from build123d import *

# Parameters (mm, degrees)
EXTRUDE_THIN1_DEPTH = 10
EXTRUDE_THIN1_DRAFT = -10
BOSS_EXTRUDE1_DEPTH = 2
CUT_EXTRUDE1_DEPTH  = 8.123412895
CIRPATTERN1_COUNT   = 4
CUT_EXTRUDE2_DEPTH  = 8.123412895
CIRPATTERN2_COUNT   = 4


with BuildPart() as part:
    # Sketch1 → Extrude-Thin1 (with draft: the straight prism first)
    with BuildSketch(Plane(origin=(0, 0, 0), x_dir=(1, 0, 0), z_dir=(0, 1, 0))):
        with BuildLine():
            ThreePointArc((22.190349254, 3.72), (15.909902577, 15.909902577), (3.72, 22.190349254))
            Line((3.72, 22.190349254), (3.72, 26.21))
            ThreePointArc((3.72, 26.21), (0, 29.93), (-3.72, 26.21))
            Line((-3.72, 26.21), (-3.72, 22.190349254))
            ThreePointArc((-3.72, 22.190349254), (-15.909902577, 15.909902577), (-22.190349254, 3.72))
            Line((-22.190349254, 3.72), (-26.21, 3.72))
            ThreePointArc((-26.21, 3.72), (-29.93, 0), (-26.21, -3.72))
            Line((-26.21, -3.72), (-22.190349254, -3.72))
            ThreePointArc((-22.190349254, -3.72), (-15.909902577, -15.909902577), (-3.72, -22.190349254))
            Line((-3.72, -22.190349254), (-3.72, -26.21))
            ThreePointArc((-3.72, -26.21), (0, -29.93), (3.72, -26.21))
            Line((3.72, -26.21), (3.72, -22.190349254))
            ThreePointArc((3.72, -22.190349254), (15.909902577, -15.909902577), (22.190349254, -3.72))
            Line((22.190349254, -3.72), (26.21, -3.72))
            ThreePointArc((26.21, -3.72), (29.93, 0), (26.21, 3.72))
            Line((26.21, 3.72), (22.190349254, 3.72))
        make_face()
        with BuildLine():
            Line((20.909289801, 2.25), (26.21, 2.25))
            ThreePointArc((26.21, 2.25), (28.46, 0), (26.21, -2.25))
            Line((26.21, -2.25), (20.909289801, -2.25))
            ThreePointArc((20.909289801, -2.25), (14.870455608, -14.870455608), (2.25, -20.909289801))
            Line((2.25, -20.909289801), (2.25, -26.21))
            ThreePointArc((2.25, -26.21), (0, -28.46), (-2.25, -26.21))
            Line((-2.25, -26.21), (-2.25, -20.909289801))
            ThreePointArc((-2.25, -20.909289801), (-14.870455608, -14.870455608), (-20.909289801, -2.25))
            Line((-20.909289801, -2.25), (-26.21, -2.25))
            ThreePointArc((-26.21, -2.25), (-28.46, 0), (-26.21, 2.25))
            Line((-26.21, 2.25), (-20.909289801, 2.25))
            ThreePointArc((-20.909289801, 2.25), (-14.870455608, 14.870455608), (-2.25, 20.909289801))
            Line((-2.25, 20.909289801), (-2.25, 26.21))
            ThreePointArc((-2.25, 26.21), (0, 28.46), (2.25, 26.21))
            Line((2.25, 26.21), (2.25, 20.909289801))
            ThreePointArc((2.25, 20.909289801), (14.870455608, 14.870455608), (20.909289801, 2.25))
        make_face(mode=Mode.SUBTRACT)
    extrude(amount=EXTRUDE_THIN1_DEPTH)
    # Extrude-Thin1: the draft: its side faces are tilted about the plane it starts from
    extrude_thin1_sides = [part.faces().sort_by_distance(p)[0] for p in [
        (-3.72, 5, 24.200174627),
        (0, 5, 29.93),
        (3.72, 5, 24.200174627),
        (15.909902577, 5, 15.909902577),
        (24.200174627, 5, 3.72),
        (29.93, 5, 0),
        (24.200174627, 5, -3.72),
        (15.909902577, 5, -15.909902577),
        (3.72, 5, -24.200174627),
        (0, 5, -29.93),
        (-3.72, 5, -24.200174627),
        (-15.909902577, 5, -15.909902577),
        (-24.200174627, 5, -3.72),
        (-29.93, 5, 0),
        (-24.200174627, 5, 3.72),
        (-15.909902577, 5, 15.909902577),
        (-23.559644901, 5, 2.25),
        (-28.46, 5, 0),
        (-23.559644901, 5, -2.25),
        (-14.870455608, 5, -14.870455608),
        (-2.25, 5, -23.559644901),
        (0, 5, -28.46),
        (2.25, 5, -23.559644901),
        (14.870455608, 5, -14.870455608),
        (23.559644901, 5, -2.25),
        (28.46, 5, 0),
        (23.559644901, 5, 2.25),
        (14.870455608, 5, 14.870455608),
        (2.25, 5, 23.559644901),
        (0, 5, 28.46),
        (-2.25, 5, 23.559644901),
        (-14.870455608, 5, 14.870455608),
    ]]
    draft(extrude_thin1_sides, Plane(origin=(0, 0, 0), x_dir=(1, 0, 0), z_dir=(0, 1, 0)), EXTRUDE_THIN1_DRAFT)

    # Sketch2 → Boss-Extrude1 (add)
    with BuildSketch(Plane.XZ):
        with BuildLine():
            Line((3.72, -26.21), (3.72, -22.190349254))
            ThreePointArc((3.72, -22.190349254), (15.909902577, -15.909902577), (22.190349254, -3.72))
            Line((22.190349254, -3.72), (26.21, -3.72))
            ThreePointArc((26.21, -3.72), (29.93, 0), (26.21, 3.72))
            Line((26.21, 3.72), (22.190349254, 3.72))
            ThreePointArc((22.190349254, 3.72), (15.909902577, 15.909902577), (3.72, 22.190349254))
            Line((3.72, 22.190349254), (3.72, 26.21))
            ThreePointArc((3.72, 26.21), (0, 29.93), (-3.72, 26.21))
            Line((-3.72, 26.21), (-3.72, 22.190349254))
            ThreePointArc((-3.72, 22.190349254), (-15.909902577, 15.909902577), (-22.190349254, 3.72))
            Line((-22.190349254, 3.72), (-26.21, 3.72))
            ThreePointArc((-26.21, 3.72), (-29.93, 0), (-26.21, -3.72))
            Line((-26.21, -3.72), (-22.190349254, -3.72))
            ThreePointArc((-22.190349254, -3.72), (-15.909902577, -15.909902577), (-3.72, -22.190349254))
            Line((-3.72, -22.190349254), (-3.72, -26.21))
            ThreePointArc((-3.72, -26.21), (0, -29.93), (3.72, -26.21))
        make_face()
    extrude(amount=-BOSS_EXTRUDE1_DEPTH)

    # Sketch4 → Cut-Extrude1 (cut, along a direction that is not the sketch's normal)
    with BuildSketch(Plane(origin=(0, 10, 0), x_dir=(1, 0, 0), z_dir=(0, 1, 0))):
        with BuildLine():
            Line((26.21, 3.723269807), (18.903548722, 3.723269807))
            ThreePointArc((18.903548722, 3.723269807), (19.266730193, 0), (18.903548722, -3.723269807))
            Line((18.903548722, -3.723269807), (26.21, -3.723269807))
            ThreePointArc((26.21, -3.723269807), (29.933269807, 0), (26.21, 3.723269807))
        make_face()
    cut_extrude1 = extrude(amount=-CUT_EXTRUDE1_DEPTH, dir=(0.17364817766693075, 0.984807753012208, 0), mode=Mode.SUBTRACT)

    # CirPattern1: Cut-Extrude1 ×4 about axis
    cirpattern1_axis = Axis((0, 0, 0), (0, -1, 0))
    for i in range(1, CIRPATTERN1_COUNT):
        add(cut_extrude1.rotate(cirpattern1_axis, i * 360 / CIRPATTERN1_COUNT), mode=Mode.SUBTRACT)

    # Sketch7 → Cut-Extrude2 (cut, along a direction that is not the sketch's normal)
    with BuildSketch(Plane(origin=(0, 10, 0), x_dir=(1, 0, 0), z_dir=(0, 1, 0))):
        with BuildLine():
            Line((3.723269807, 18.903548722), (3.723269807, 22.487116544))
            ThreePointArc((3.723269807, 22.487116544), (16.117275646, 16.117275646), (22.487116544, 3.723269807))
            Line((22.487116544, 3.723269807), (18.903548722, 3.723269807))
            ThreePointArc((18.903548722, 3.723269807), (13.623635571, 13.623635571), (3.723269807, 18.903548722))
        make_face()
    cut_extrude2 = extrude(amount=-CUT_EXTRUDE2_DEPTH, dir=(0.12278780396897289, 0.9848077530122081, -0.12278780396897289), mode=Mode.SUBTRACT)

    # CirPattern2: Cut-Extrude2 ×4 about axis
    cirpattern2_axis = Axis((0, 0, 0), (0, -1, 0))
    for i in range(1, CIRPATTERN2_COUNT):
        add(cut_extrude2.rotate(cirpattern2_axis, i * 360 / CIRPATTERN2_COUNT), mode=Mode.SUBTRACT)


solid = part.part
For this review, take the finished solid that the model builds, in its own axes (mm). A direction names the side the tool comes from. Give positions to 0.01 mm unless a question says otherwise; leave off trailing zeros.
Item 1: For line 1 along Y through (x, z) = (12.5, 3.5); line 2 along Z through (x, y) = (7.5, 8); line 3 along X through (y, z) = (5, 19), list the stretches that pass through material, from the lowest coordinate up.
Item 2: Tool access review of faces 4 (the flat face through (-24, 6, 3.723)), 5 (the flat face through (24.62, 4.93, 4.59)), 6 (the flat face through (-24.62, 4.93, -4.59)), 7 (the flat face through (24.67, 4.93, -4.59)): name each direction out of +Z, -Z, +X, -X, +Y, -Y from which nothing blocks a thin tool from reaching the whole face with its end or side.
Item 3: Insertion check: pin 1 (6 mm diameter, centred on x = -3.5, y = 7.5, fed in from -Z); pin 2 (1.5 mm diameter, centred on y = 6, z = -24, fed in from -X); pin 3 (1 mm diameter, centred on y = 3, z = 13.5, fed in from -X). Each pin has a flat end and moves straight along its axis. Give the tip position at first contact, or say it passes through.
Item 4: Draft analysis for pull direction X (two halves, no side actions). For faces 1 (the flat face through (0, 2, 0)), 2 (the flat face through (0, 0, 0)), 3 (the conical face through (-16.67, 4.93, 16.38)), state which applies: +X half, -X half, draft (parallel to the pull), parting line (faces both ways), or undercut.
Calculated:
1. line 1: y = 0 to 2
1. line 2: z = -22.7 to -21.19, 21.19 to 22.7
1. line 3: x = -13.63 to -10.97, 10.97 to 13.63
2. face 4: +Y
2. face 5: +Z, +X, -Y
2. face 6: -Z, -X, -Y
2. face 7: -Z, +X, -Y
3. pin 1: stops at z = -31.46
3. pin 2: stops at x = -4.91
3. pin 3: stops at x = -19.03
4. face 1: undercut
4. face 2: draft
4. face 3: -X half
